Here's how the part is built. I have some questions about the finished solid (model axes, mm). A direction names the side the tool comes from. Coordinates: 2 decimals unless noted, no trailing zeros. Write each loop counter-clockwise with the first axis right and the second up, starting at its lowest first coordinate (ties: lowest second). Pieces come first, ordered by that corner, then holes. Notation, with made-up numbers: (41.5, 65) -> (66.5, 65) arc R19 cw to (66.5, 99) -> close; hole circle Ø4 at (68, 48.25). An arc over 180 degrees is marked (long way). Put each result on its own line as item: value. Start each with the question number.
Item 1: I want a section at C-C, the plane y = -51.5. List the corners of the cut face in (x, z) for me, then the cut area to 3 significant figures.
Item 2: I want a section at A-A, the plane y = 4. List the corners of the cut face in (x, z) for me.
Item 3: On a 3-axis mill with a long thin cutter (end or side, diameter ignored), from which of +Z, -Z, +X, -X, +Y, -Y can I reach the whole of each face in a straight line? I mean faces 1 (the face through (-0.54, -31.31, 2.44)), 2 (the face through (1.5, 8.44, 0.07)), 3 (the face through (-6, 3, 0)). Say none if no direction works.
Item 4: For pin 1 (1.5 mm diameter, centred on y = -15.5, z = 2.5, fed in from +X); pin 2 (3 mm diameter, centred on y = -11.5, z = 3.5, fed in from +X); pin 3 (3 mm diameter, centred on y = -13, z = 1.5, fed in from -X); pin 4 (5 mm diameter, centred on x = 0, y = 4, fed in from -Z), each with a flat end and sliding along its axis, tell me the tip position at first contact or that it passes through.
Item 5: If we mould it in two halves opening along X, with no side actions, what happens to faces 4 (the face through (6, 3, 0)), 5 (the face through (0, 2, 0)), 6 (the face through (1, 6, 5))? For each: released by +X, released by -X, zero draft, split by the parting line, or undercut.
Item 6: I want a section at B-B, the plane x = 0. State how many separate pieces and enclosed holes the cut face has, then the cut area to 3 significant figures.
Item 7: I need wall thicknesses on line 1 (X direction, y = -2, z = 1.5); line 2 (Y direction, x = 0.5, z = -3.75); line 3 (X direction, y = -16.5, z = -0.25). Which ranges of each line are inside material? Lowest first, please. Write a range as [from, to].
Autodesk Inventor part; units mm, degrees
ref_plane "Work Plane1" through (0, 11.5, 0) normal (0, 1, 0) x (-1, 0, 0)
ref_plane "YZ Plane" through (0, 0, 0) normal (1, 0, 0) x (0, 1, 0)
ref_plane "XY Plane" through (0, 0, 0) normal (0, 0, 1) x (1, 0, 0)
sketch "Sketch1" plane through (0, 0, 0) normal (0, 1, 0) x (-1, 0, 0)
  circle A0 centre (0, 0) radius 6
  dimension "d0" = 12
extrude "Extrusion1" add sketch "Sketch1" along normal blind 11.5
fillet "Fillet1" radius 5 1 edges at (6, 11.5, 0)
sketch "Sketch2" plane through (0, 0, 0) normal (0, -1, 0) x (1, 0, 0)
  circle A0 centre (0, 0) radius 2.5
  dimension "d4" = 5
extrude "Extrusion2" add sketch "Sketch2" along normal blind 63.5
sketch "Sketch3" plane through (0, 0, 0) normal (0, -1, 0) x (1, 0, 0)
  circle A0 centre (0, 0) radius 2.5 construction
  line L0 (0, -5) -> (0, 5) construction
  circle A1 centre (0, 0) radius 6
  line L1 (-3.3166, -5) -> (3.3166, -5)
  line L2 (-3.3166, 5) -> (3.3166, 5)
  dimension "d8" = 10
extrude "Extrusion3" cut sketch "Sketch3" against normal through all contours L2 A1 | A1 L1
sketch "Sketch4" plane through (3.3166, 0, -5) normal (0, 0, -1) x (-1, 0, 0)
  line L0 (3.3166, 0) -> (3.3166, 4) construction
  circle A0 centre (3.3166, 4) radius 2
  dimension "d11" = 4
extrude "Extrusion4" cut sketch "Sketch4" against normal through all
ref_plane "Work Plane1" through (0, 11.5, 0) normal (0, 1, 0) x (-1, 0, 0)
sketch "Sketch5" plane through (0, 11.5, 0) normal (0, 1, 0) x (-1, 0, 0)
  circle A0 centre (0, 0) radius 1.5
extrude "Extrusion5" cut sketch "Sketch5" against normal up to surface
properties part number "Asta cassetto"
Calculated:
1. outline: circle Ø5 at (0, 0)
1. area: 19.6 mm2
2. outline: (-3.32, -5) -> (-2, -5) -> (-2, 5) -> (-3.32, 5) arc R6 ccw to start; (2, -5) -> (3.32, -5) arc R6 ccw to (3.32, 5) -> (2, 5) -> close
3. face 1: -Y
3. face 2: +Y
3. face 3: -X, +Y, -Y
4. pin 1: stops at x = 1.79
4. pin 2: stops at x = 1.5
4. pin 3: stops at x = -2.5
4. pin 4: stops at z = -5
5. face 4: released by +X
5. face 5: undercut
5. face 6: zero draft
6. separate pieces: 3
6. enclosed holes: 0
6. area: 371 mm2
7. line 1: x = [-2, 2]
7. line 2: y = [0, 2.06], [5.94, 10.65]
7. line 3: x = [-2.49, 2.49]
